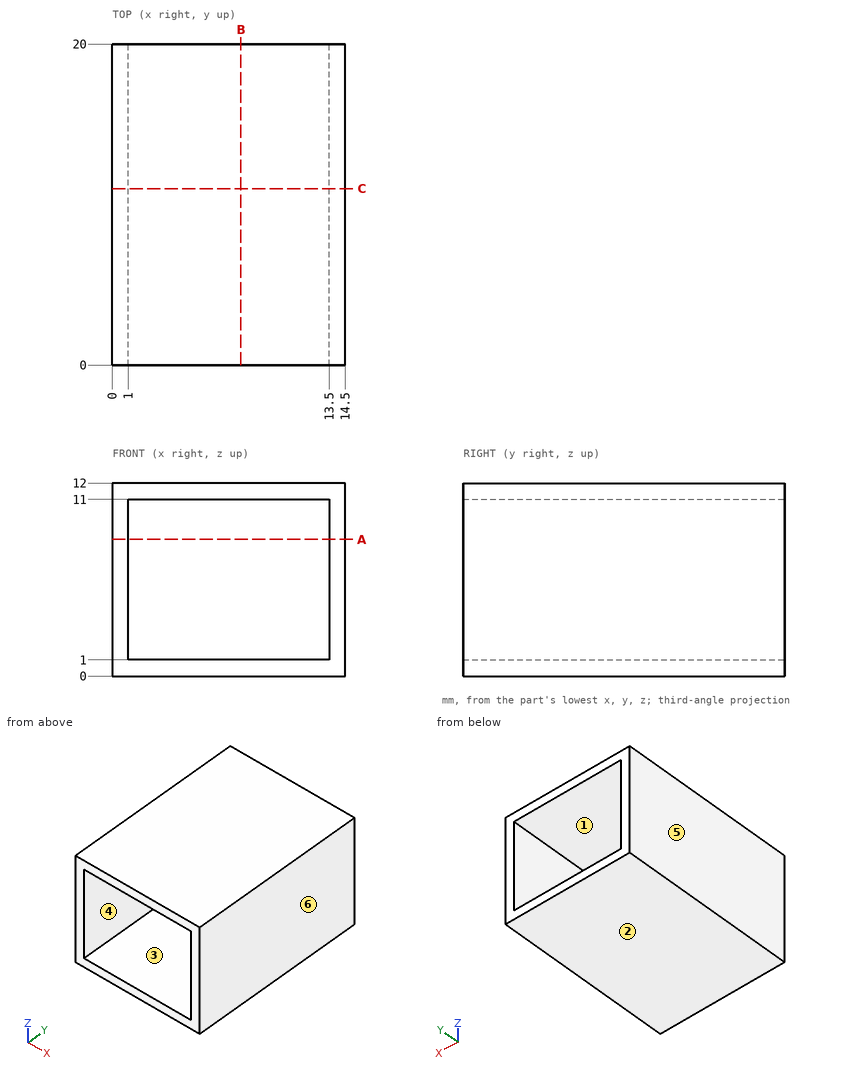
Design review of the part shown in the three views and the two pictorial views. Dimensions are in mm from the part's minimum x, y and z. A direction names the side the tool comes from. Coordinates: 2 decimals unless noted, no trailing zeros. Order: outer loops, then holes, each group sorted by start corner. A loop starts at its lowest first (then second) coordinate and runs counter-clockwise, first axis right, second up. Notation, with made-up numbers: (-28.5, 69) -> (15.5, 69) arc R21 cw to (15.5, 104) -> close; hole circle Ø11 at (61, 42). An arc over 180 degrees is marked (long way). Use one line per item in the form item = value. Start each with the question number.
(1) For probe 1 along X at (y, z) = (19, 6.75); probe 2 along Z at (x, y) = (3, 1.75), list the stretches that pass through material, from the lowest coordinate up.
(2) Add section B-B on x = 8. State the section outline as (y, z) points, plus the area to 3 significant figures.
(3) Add section A-A on z = 8.5. State the section outline as (x, y) points.
(4) For the marked faces 1 and 2, list the 3-axis set-ups (+Z, -Z, +X, -X, +Y, -Y) from which the entire face can be reached by the end or side of a thin tool; tool diameter is ignored.
(5) The part is to be moulded in two halves that separate along X. For the marked faces 3, 4, 5 and 6, say which applies: +X half, -X half, draft (parallel to the pull), parting line (faces both ways), or undercut.
(6) Insertion check: pin 1 (5 mm diameter, centred on x = 13, z = 5.5, fed in from +Y); pin 2 (1 mm diameter, centred on x = 3, z = 2, fed in from +Y). Each pin has a flat end and moves straight along its axis. Give the tip position at first contact, or say it passes through.
(7) Add section C-C on y = 11. State the section outline as (x, z) points, plus the area to 3 significant figures.
Answer block:
q1.probe_1 = 0 to 1, 13.5 to 14.5
q1.probe_2 = 0 to 1, 11 to 12
q2.outline = (0, 0) -> (20, 0) -> (20, 1) -> (0, 1) -> close; (0, 11) -> (20, 11) -> (20, 12) -> (0, 12) -> close
q2.area = 40.0 mm²
q3.outline = (0, 0) -> (1, 0) -> (1, 20) -> (0, 20) -> close; (13.5, 0) -> (14.5, 0) -> (14.5, 20) -> (13.5, 20) -> close
q4.face_1 = +Y, -Y
q4.face_2 = -Z, +X, -X, +Y, -Y
q5.face_3 = undercut
q5.face_4 = undercut
q5.face_5 = -X half
q5.face_6 = +X half
q6.pin_1 = 20
q6.pin_2 = through
q7.outline = (0, 0) -> (14.5, 0) -> (14.5, 12) -> (0, 12) -> close; hole (1, 1) -> (13.5, 1) -> (13.5, 11) -> (1, 11) -> close
q7.area = 49.0 mm²
